```python
from build123d import *

# Parameters (mm, degrees)
SKETCH1_W                   = 147.5
SKETCH1_H                   = 210
BOSS_EXTRUDE1_DEPTH         = 2
SKETCH3_W                   = 25
SKETCH3_H                   = 12.7
BOSS_EXTRUDE3_DEPTH         = 4
M4_TAPPED_HOLE1_D           = 3.3
M4_TAPPED_HOLE1_CSINK_D     = 4.05
M4_TAPPED_HOLE1_CSINK_ANGLE = 90


with BuildPart() as part:
    # Sketch1 → Boss-Extrude1 (new body)
    with BuildSketch(Plane(origin=(0, 0, 0), x_dir=(1, 0, 0), z_dir=(0, 1, 0))):
        Rectangle(SKETCH1_W, SKETCH1_H)
    extrude(amount=BOSS_EXTRUDE1_DEPTH)

    # Sketch3 → Boss-Extrude3 (add)
    with BuildSketch(Plane(origin=(0, 2, 0), x_dir=(1, 0, 0), z_dir=(0, 1, 0))):
        with Locations((-27.5, 0)):
            Rectangle(SKETCH3_W, SKETCH3_H)
    extrude(amount=BOSS_EXTRUDE3_DEPTH)

    # M4 Tapped Hole1 (through all)
    with Locations(Plane(origin=(0, 6, 0), x_dir=(1, 0, 0), z_dir=(0, 1, 0))):
        with Locations((-20, 0), (-35, 0)):
            CounterSinkHole(M4_TAPPED_HOLE1_D / 2, M4_TAPPED_HOLE1_CSINK_D / 2, counter_sink_angle=M4_TAPPED_HOLE1_CSINK_ANGLE)


solid = part.part
```
The model under review builds one solid part; all positions refer to its coordinate system, in mm. A direction names the side the tool comes from. Give positions to 0.01 mm unless a question says otherwise; leave off trailing zeros. Write each loop counter-clockwise with the first axis right and the second up, starting at its lowest first coordinate (ties: lowest second). Pieces come first, ordered by that corner, then holes. Notation, with made-up numbers: (88, 48) -> (93, 48) arc R17 cw to (93, 69) -> close; hole circle Ø1 at (73, 50). An arc over 180 degrees is marked (long way). Answer in a Markdown table with one row per item.
1) Tool access review of faces 1 (the flat face through (-40, 4, 0)), 2 (the flat face through (-28, 4, 6.35)), 3 (the flat face through (-15, 4, 0)): name each direction out of +Z, -Z, +X, -X, +Y, -Y from which nothing blocks a thin tool from reaching the whole face with its end or side.
Worked answers:
| item | result |
|---|---|
| face 1 | +Z, -Z, -X, +Y |
| face 2 | +Z, +X, -X, +Y |
| face 3 | +Z, -Z, +X, +Y |
2) Add section A-A on y = 3.4. State the section outline as (x, z) points.
Worked answers:
| item | result |
|---|---|
| outline | (-40, -6.35) -> (-15, -6.35) -> (-15, 6.35) -> (-40, 6.35) -> close; hole circle Ø3.3 at (-35, 0); hole circle Ø3.3 at (-20, 0) |
3) Add section B-B on x = -24.5. State the section outline as (y, z) points, plus the area to 3 significant figures.
Worked answers:
| item | result |
|---|---|
| outline | (0, -105) -> (2, -105) -> (2, -6.35) -> (6, -6.35) -> (6, 6.35) -> (2, 6.35) -> (2, 105) -> (0, 105) -> close |
| area | 471 mm² |
4) Clearance check with flat-ended pins moving along their axes: P1, Ø1.2, axis at y = 3.5, z = 3, coming from the +X side; P2, Ø1.5, axis at x = -9, y = 4.5, coming from the +Z side; P3, Ø1.2, axis at x = -31, y = 4, coming from the -Z side; P4, Ø4, axis at x = -20, z = 0, coming from the +Y side (3 decimals). State where each tip first meets the part, or that it passes through.
Worked answers:
| item | result |
|---|---|
| P1 | x = -15 |
| P2 | through |
| P3 | z = -6.35 |
| P4 | y = 5.975 |
5) Add section D-D on x = 27. State the section outline as (y, z) points, plus the area to 3 significant figures.
Worked answers:
| item | result |
|---|---|
| outline | (0, -105) -> (2, -105) -> (2, 105) -> (0, 105) -> close |
| area | 420 mm² |
6) For L1, parallel to Z at x = -35, y = 3.9; L2, parallel to Z at x = -20, y = 1.7; L3, parallel to Y at x = 65, z = 21, list the stretches that pass through material, from the lowest coordinate up. Write a range as [from, to].
Worked answers:
| item | result |
|---|---|
| L1 | [-6.35, -1.65], [1.65, 6.35] |
| L2 | [-105, -1.65], [1.65, 105] |
| L3 | [0, 2] |
7) Add section C-C on z = -27. State the section outline as (x, y) points.
Worked answers:
| item | result |
|---|---|
| outline | (-73.75, 0) -> (73.75, 0) -> (73.75, 2) -> (-73.75, 2) -> close |
